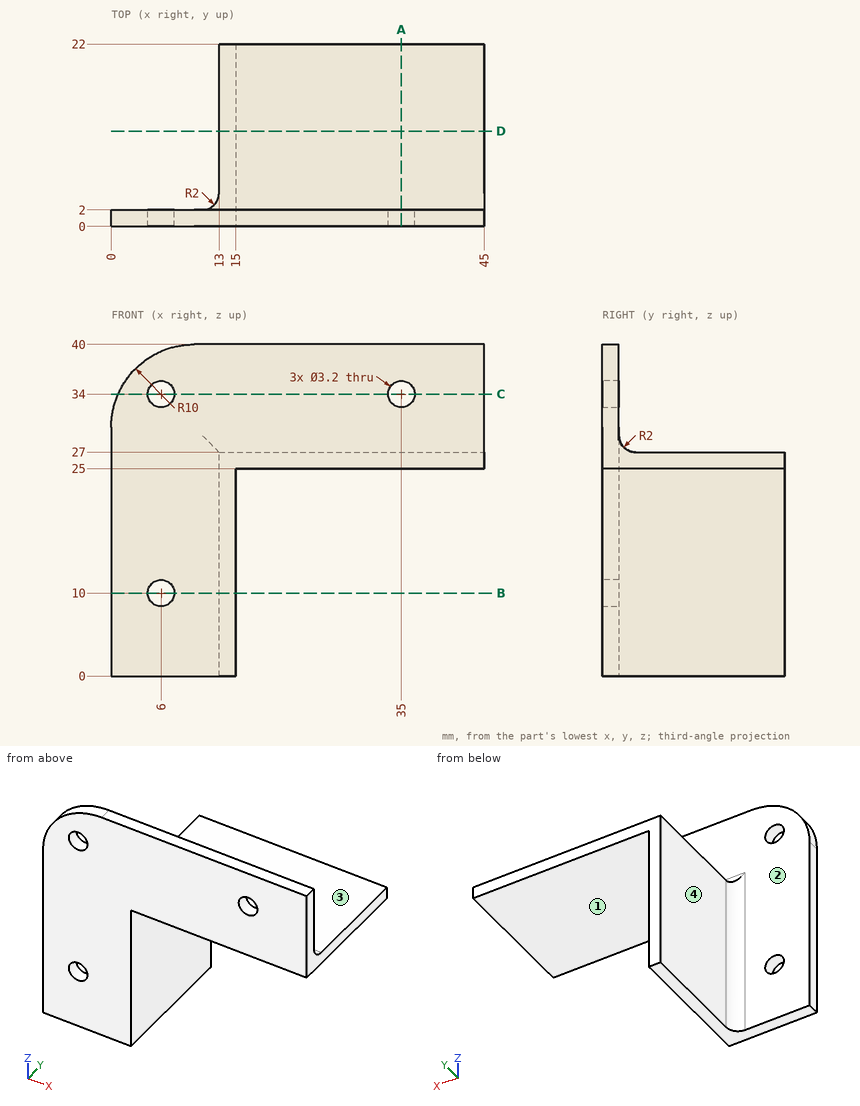
Input: dimensioned drawing with shaded views. Units: mm. Origin: part minimum x, y, z. A direction names the side the tool comes from. Give positions to 0.01 mm unless a question says otherwise; leave off trailing zeros. Write each loop counter-clockwise with the first axis right and the second up, starting at its lowest first coordinate (ties: lowest second). Pieces come first, ordered by that corner, then holes. Notation, with made-up numbers: (88.25, 53.5) - (131.25, 53.5) arc R17 cw to (131.25, 63.5) - close; hole circle Ø2 at (-2.75, 4). An arc over 180 degrees is marked (long way). One line per item, written item: value. Start each with the question number.
Q1. First-contact query: pin 1 Ø2 at (x, y) = (36.5, 6) entering from +Z; pin 2 Ø1 at (y, z) = (3.5, 18) entering from -X; pin 3 Ø3 at (x, z) = (6, 10) entering from +Y; pin 4 Ø12 at (y, z) = (12.5, 21.5) entering from -X. Flat tips, straight axial feed; report the tip coordinate or a pass-through.
Q2. Section query A-A, the plane x = 35. Return the cut outline in (y, z), then the cut area to 3 significant figures.
Q3. Section query D-D, the plane y = 11.5. Return the cut outline in (x, z), then the cut area to 3 significant figures.
Q4. Material intervals for probe 1 along X at (y, z) = (1.05, 34); probe 2 along X at (y, z) = (1.2, 10); probe 3 along Y at (x, z) = (30.5, 32), sorted ascending. Write a range as from..to.
Q5. Section query C-C, the plane z = 34. Return the cut outline in (x, y), then the cut area to 3 significant figures.
Q6. Section query B-B, the plane z = 10. Return the cut outline in (x, y), then the cut area to 3 significant figures.
Q7. Set-up query: the marked faces 1, 2, 3 and 4. Return all of +Z, -Z, +X, -X, +Y, -Y with unobstructed straight access to the full face (end or side cutting, diameter ignored); none if empty.
Answer:
1. pin 1: stops at z = 27
1. pin 2: stops at x = 12.73
1. pin 3: passes through
1. pin 4: stops at x = 13
2. outline: (0, 25) - (22, 25) - (22, 27) - (4, 27) arc R2 cw to (2, 29) - (2, 32.4) - (0, 32.4) - close; (0, 35.6) - (2, 35.6) - (2, 40) - (0, 40) - close
2. area: 64.5 mm2
3. outline: (13, 0) - (15, 0) - (15, 25) - (45, 25) - (45, 27) - (13, 27) - close
3. area: 114 mm2
4. probe 1: x = 0.83..4.4, 7.6..33.4, 36.6..45
4. probe 2: x = 0..4.4, 7.6..15
4. probe 3: y = 0..2
5. outline: (0.83, 0) - (4.4, 0) - (4.4, 2) - (0.83, 2) - close; (7.6, 0) - (33.4, 0) - (33.4, 2) - (7.6, 2) - close; (36.6, 0) - (45, 0) - (45, 2) - (36.6, 2) - close
5. area: 75.5 mm2
6. outline: (0, 0) - (4.4, 0) - (4.4, 2) - (0, 2) - close; (7.6, 0) - (15, 0) - (15, 22) - (13, 22) - (13, 4) arc R2 cw to (11, 2) - (7.6, 2) - close
6. area: 64.5 mm2
7. face 1: -Z, +X, +Y, -Y
7. face 2: +Z, -X, +Y
7. face 3: +Z, +X, -X, +Y
7. face 4: +Z, -Z, -X, +Y
